Can you work these out from the model? Positions are in its coordinate system, mm. A direction names the side the tool comes from. Round coordinates to 2 decimals unless told otherwise and drop trailing zeros. Loops run counter-clockwise (first coordinate to the right, second up) from the corner with the lowest first, then second, coordinate; pieces in that order, holes last. Notation, with made-up numbers: M -23,36.5 L 19,36.5 A23 cw 19,63.5 Z; hole C -31,-26.75 d8. An arc over 180 degrees is marked long. Return JSON: item names as keys, results as strings.
```python
from build123d import *

# Parameters (mm, degrees)
SKETCH1_W            = 90
SKETCH1_H            = 27.5
BOSS_EXTRUDE1_DEPTH  = 10
CUT_EXTRUDE1_DEPTH   = 28.5
SKETCH9_W            = 40
SKETCH9_H            = 40
BOSS_EXTRUDE3_DEPTH  = 10
CUT_EXTRUDE2_DEPTH   = 2
M4_CLEARANCE_HOLE1_D = 4.5
FILLET1_R            = 5
SKETCH10_R           = 2
CUT_EXTRUDE3_DEPTH   = 11


with BuildPart() as part:
    # Sketch1 → Boss-Extrude1 (new body)
    with BuildSketch(Plane(origin=(0, 0, 0), x_dir=(1, 0, 0), z_dir=(0, 1, 0))):
        with Locations((-45, 13.75)):
            Rectangle(SKETCH1_W, SKETCH1_H)
    extrude(amount=BOSS_EXTRUDE1_DEPTH)

    # Sketch2 → Cut-Extrude1 (cut, through all)
    with BuildSketch(Plane.XY):
        Polygon((-32.4, 3.4988893), (-32.4, 6.5011107), (-35, 8.0022214), (-37.6, 6.5011107), (-37.6, 3.4988893), (-35, 1.9977786), align=None)
        Polygon((-2.4, 3.4988893), (-2.4, 6.5011107), (-5, 8.0022214), (-7.6, 6.5011107), (-7.6, 3.4988893), (-5, 1.9977786), align=None)
    extrude(amount=-CUT_EXTRUDE1_DEPTH, mode=Mode.SUBTRACT)

    # Sketch9 → Boss-Extrude3 (add)
    with BuildSketch(Plane(origin=(0, 10, 0), x_dir=(1, 0, 0), z_dir=(0, 1, 0))):
        with Locations((-70, 7.5)):
            Rectangle(SKETCH9_W, SKETCH9_H)
    extrude(amount=-BOSS_EXTRUDE3_DEPTH)

    # Sketch4 → Cut-Extrude2 (cut)
    with BuildSketch(Plane(origin=(-50, 10, 0), x_dir=(0, 0, -1), z_dir=(0, 1, 0))):
        Polygon((27.6, 44.841124336), (27.6, 37.258569022), (27.6, 14.504295037), (24.6, 14.504295037), (24.6, 37.289189868), (21.85, 37.289189868), (21.85, 30.489189868), (21.85, 14.289189868), (9.45, 14.289189868), (9.45, 30.489189868), (9.45, 37.289189868), (5.65, 37.289189868), (5.65, 30.489189868), (5.65, 14.289189868), (-6.75, 14.289189868), (-6.75, 30.489189868), (-6.75, 37.289189868), (-9.5, 37.289189868), (-9.5, 14.289189868), (-12.5, 14.289189868), (-12.5, 37.289189868), (-12.5, 44.841124336), align=None)
    extrude(amount=-CUT_EXTRUDE2_DEPTH, mode=Mode.SUBTRACT)

    # M4 Clearance Hole1 (through all)
    with Locations(Plane(origin=(0, 8, 0), x_dir=(0, 0, -1), z_dir=(0, 1, 0))):
        with Locations((-0.35, 74.289189868), (15.45, 74.289189868)):
            Hole(M4_CLEARANCE_HOLE1_D / 2)

    # Fillet1
    fillet1_edges = [part.edges().sort_by_distance(p)[0] for p in [
        (-90, 4, 12.5),
        (-50, 5, 0),
        (-50, 5, 12.5),
        (-90, 4, -27.5),
    ]]
    fillet(fillet1_edges, radius=FILLET1_R)

    # Sketch10 → Cut-Extrude3 (cut, through all)
    with BuildSketch(Plane(origin=(0, 10, 0), x_dir=(1, 0, 0), z_dir=(0, 1, 0))):
        with Locations((-19.5, 4.106184291)):
            Circle(SKETCH10_R)
        with Locations((-19.5, 22.106184291)):
            Circle(SKETCH10_R)
        with BuildLine():
            Line((-17, 8.106184291), (-22, 8.106184291))
            ThreePointArc((-22, 8.106184291), (-27, 13.106184291), (-22, 18.106184291))
            Line((-22, 18.106184291), (-17, 18.106184291))
            ThreePointArc((-17, 18.106184291), (-12, 13.106184291), (-17, 8.106184291))
        make_face()
    extrude(amount=-CUT_EXTRUDE3_DEPTH, mode=Mode.SUBTRACT)


solid = part.part
```
Q1. I'm going to push flat-ended pins straight in: pin 1 Ø1.6 at (y, z) = (9.5, 3.5) entering from -X; pin 2 Ø3 at (x, y) = (-28.5, 5) entering from +Z; pin 3 Ø1.6 at (x, y) = (-72.5, 9) entering from +Z; pin 4 Ø2.5 at (x, z) = (-74.29, 0.35) entering from +Y. Where does each tip first touch, or does it pass through?
Results:
{"pin 1": "stops at x = -64.29", "pin 2": "stops at z = 0", "pin 3": "stops at z = 9.5", "pin 4": "passes through"}
Q2. On a 3-axis mill with a long thin cutter (end or side, diameter ignored), from which of +Z, -Z, +X, -X, +Y, -Y can I reach the whole of each face in a straight line? I mean faces 1 (the flat face through (-23, 5, 0)), 2 (the flat face through (-76, 9, 6.75)), 3 (the flat face through (-87.289, 9, -23)), 4 (the flat face through (-33.68, 7.24, -13.56)). Say none if no direction works.
Results:
{"face 1": "+Z, +X, +Y, -Y", "face 2": "-X, +Y", "face 3": "+Z, -Z, -X, +Y", "face 4": "+Z, -Z"}
Q3. Thinking about a two-plate mould opening in Z: for faces 5 (the flat face through (-76, 9, -5.65)), 6 (the cylindrical face through (-20.97, 5.07, -5.46)), 7 (the cylindrical face through (-51.5, 4.93, 11.07)), 8 (the flat face through (-56, 0, -12)), which applies, pulls with the +Z half, pulls with the -Z half, needs draft (parallel to the pull), parting line crosses it, or undercut?
Results:
{"face 5": "undercut", "face 6": "undercut", "face 7": "pulls with the +Z half", "face 8": "needs draft"}
Q4. Suppose I cut it at B-B, the plane x = -70. Please give me the cut outline in (y, z).
Results:
{"outline": "M 0,-27.5 L 8,-27.5 L 8,-24.6 L 10,-24.6 L 10,-21.85 L 8,-21.85 L 8,-9.45 L 10,-9.45 L 10,-5.65 L 8,-5.65 L 8,6.75 L 10,6.75 L 10,9.5 L 8,9.5 L 8,12.5 L 0,12.5 Z"}
Q5. Suppose I cut it at C-C, the plane z = -15.45. Please give me the cut outline in (x, y).
Results:
{"outline": "M -90,0 L -76.54,0 L -76.54,8 L -90,8 Z; M -72.04,0 L -26.42,0 L -26.42,10 L -64.29,10 L -64.29,8 L -72.04,8 Z; M -12.58,0 L 0,0 L 0,10 L -12.58,10 Z; hole M -37.6,3.5 L -35,2 L -32.4,3.5 L -32.4,6.5 L -35,8 L -37.6,6.5 Z; hole M -7.6,3.5 L -5,2 L -2.4,3.5 L -2.4,6.5 L -5,8 L -7.6,6.5 Z"}
Q6. Suppose I cut it at A-A, the plane y = 5.5. Please give me the cut outline in (x, z), plus the area to 3 significant figures.
Results:
{"outline": "M -90,-22.5 A5 ccw -85,-27.5 L -37.6,-27.5 L -37.6,0 L -45,0 A5 cw -50,5 L -50,7.5 A5 ccw -55,12.5 L -85,12.5 A5 ccw -90,7.5 Z; M -32.4,-27.5 L -7.6,-27.5 L -7.6,0 L -32.4,0 Z; M -2.4,-27.5 L 0,-27.5 L 0,0 L -2.4,0 Z; hole C -74.29,-15.45 d4.5; hole C -74.29,0.35 d4.5; hole M -22,-18.11 L -17,-18.11 A5 ccw -17,-8.11 L -22,-8.11 A5 ccw Z; hole C -19.5,-22.11 d4; hole C -19.5,-4.11 d4", "area": "2,490 mm2"}
Q7. Suppose I cut it at D-D, the plane x = -36.5. Please give me the cut outline in (y, z).
Results:
{"outline": "M 0,-27.5 L 2.86,-27.5 L 2.86,0 L 0,0 Z; M 7.14,-27.5 L 10,-27.5 L 10,0 L 7.14,0 Z"}
Q8. If I drill on line 1 along Z through (x, y) = (-19.5, 5.5); line 2 along X through (y, z) = (5, -19); line 3 along Z through (x, y) = (-76, 6.25), over which ranges is the centre line in solid material (lowest first)?
Results:
{"line 1": "z = -27.5 to -24.11, -20.11 to -18.11, -8.11 to -6.11, -2.11 to 0", "line 2": "x = -90 to -37.6, -32.4 to -7.6, -2.4 to 0", "line 3": "z = -27.5 to -16.91, -13.99 to -1.11, 1.81 to 12.5"}
